Work out the finished part from the listing and answer in its coordinate system (mm). Face numbers are marked on the shaded views. A direction names the side the tool comes from. Round coordinates to 2 decimals unless told otherwise and drop trailing zeros. Order: outer loops, then holes, each group sorted by start corner. A loop starts at its lowest first (then second) coordinate and runs counter-clockwise, first axis right, second up. Notation, with made-up numbers: (79, -26) - (99, -26) arc R22 cw to (99, -6) - close; hole circle Ø1 at (28.5, 19.25). An arc over 180 degrees is marked (long way). Use CSV: the item, a comma, the result in double quotes.
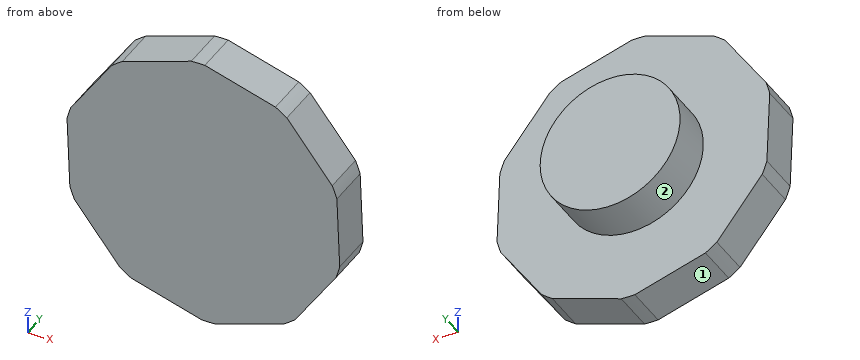
from build123d import *

# Parameters (mm, degrees)
F0_R     = 5
F1_DEPTH = 3
F2_R     = 10
F3_DEPTH = 3
F4_R     = 11.267003
F5_DEPTH = 25


with BuildPart() as f1:
    # F0 (on Front) → F1 (new body)
    with BuildSketch(Plane.XZ):
        Circle(F0_R)
    extrude(amount=F1_DEPTH)

    # F2 (on face) → F3 (join)
    with BuildSketch(Plane.XZ.offset(3)):
        Circle(F2_R)
    extrude(amount=F3_DEPTH)

    # F4 (on face) → F5 (cut)
    with BuildSketch(Plane.XZ.offset(6)):
        Circle(F4_R)
        Polygon((-6.271795, 7.976108), (-0.38575, 10.139275), (5.647638, 8.429584), (9.52382, 3.500078), (9.762227, -2.766338), (6.271795, -7.976108), (0.38575, -10.139275), (-5.647638, -8.429584), (-9.52382, -3.500078), (-9.762227, 2.766338), align=None, mode=Mode.SUBTRACT)
    extrude(amount=-F5_DEPTH, mode=Mode.SUBTRACT)


solid = f1.part
(1) Find section C-C (x = -2.5). Determine the outline of the cut face in (y, z), and give its area (3 significant figures).
Findings below:
outline,"(-6, -9.32) - (-3, -9.32) - (-3, -4.33) - (0, -4.33) - (0, 4.33) - (-3, 4.33) - (-3, 9.36) - (-6, 9.36) - close"
area,"82.0 mm²"
(2) Find section B-B (y = -4.4). Determine the outline of the cut face in (x, z).
Findings below:
outline,"(-9.74, 2.25) - (-9.54, -2.99) arc R10 ccw to (-9.21, -3.9) - (-5.96, -8.03) arc R10 ccw to (-5.15, -8.57) - (-0.11, -10) arc R10 ccw to (0.87, -9.96) - (5.79, -8.15) arc R10 ccw to (6.56, -7.55) - (9.48, -3.19) arc R10 ccw to (9.74, -2.25) - (9.54, 2.99) arc R10 ccw to (9.21, 3.9) - (5.96, 8.03) arc R10 ccw to (5.15, 8.57) - (0.11, 10) arc R10 ccw to (-0.87, 9.96) - (-5.79, 8.15) arc R10 ccw to (-6.56, 7.55) - (-9.48, 3.19) arc R10 ccw to start"
(3) For the marked faces 1 and 2, determine the directions among +Z, -Z, +X, -X, +Y, -Y from which every point of the face is accessible in a straight line to the end or side of a thin tool.
Findings below:
face 1,"-Z, -X, +Y, -Y"
face 2,"+Y"
(4) Find section D-D (y = -2.45). Determine the outline of the cut face in (x, z).
Findings below:
outline,"circle Ø10 at (0, 0)"
(5) Each of these flat-tipped pins is pushed along its axis until it touches: pin 1 (3 mm diameter, centred on y = -1, z = 7.5, fed in from +X); pin 2 (2 mm diameter, centred on x = -4, y = -5.5, fed in from -Z). Where does it stop, or does it pass through?
Findings below:
pin 1,"passes through"
pin 2,"stops at z = -9.18"
(6) Find the intervals of material crossed by L1, parallel to Y at x = 8.75, z = 0.25; L2, parallel to X at y = -4.2, z = 4.5; L3, parallel to X at y = -2.2, z = -3, in increasing order. Write a range as from..to.
Findings below:
L1,"y = -6..-3"
L2,"x = -8.6..8.74"
L3,"x = -4..4"
(7) Find section A-A (z = 0). Determine the outline of the cut face in (x, y), and give its area (3 significant figures).
Findings below:
outline,"(-9.66, -6) - (9.66, -6) - (9.66, -3) - (5, -3) - (5, 0) - (-5, 0) - (-5, -3) - (-9.66, -3) - close"
area,"87.9 mm²"
